```python
from build123d import *

# Parameters (mm, degrees)
SKETCH2_W            = 100
SKETCH2_H            = 100
BOSS_EXTRUDE1_DEPTH  = 5
SKETCH3_W            = 100
SKETCH3_H            = 100
BOSS_EXTRUDE2_DEPTH  = 5
SKETCH8_R            = 5
BOSS_EXTRUDE7_DEPTH  = 30
SKETCH9_W            = 35.4
SKETCH9_H            = 35.4
BOSS_EXTRUDE8_DEPTH  = 20
SKETCH10_W           = 25.4
SKETCH10_H           = 25.4
CUT_EXTRUDE1_DEPTH   = 12.7
BOSS_EXTRUDE21_DEPTH = 10
FILLET14_R           = 4
FILLET13_R           = 4
SKETCH24_W           = 10
SKETCH24_H           = 10
BOSS_EXTRUDE22_DEPTH = 15
BOSS_EXTRUDE25_DEPTH = 10
SKETCH26_W           = 10
SKETCH26_H           = 10
BOSS_EXTRUDE26_DEPTH = 15
FILLET18_R           = 4
FILLET17_R           = 4
BOSS_EXTRUDE23_DEPTH = 10
SKETCH25_W           = 10
SKETCH25_H           = 10
BOSS_EXTRUDE24_DEPTH = 15
FILLET15_R           = 4
FILLET16_R           = 4
BOSS_EXTRUDE10_DEPTH = 10
FILLET19_R           = 4
SKETCH27_W           = 10
SKETCH27_H           = 10
BOSS_EXTRUDE27_DEPTH = 15
FILLET20_R           = 4
SKETCH33_W           = 65
SKETCH33_H           = 65
BOSS_EXTRUDE29_DEPTH = 5
BOSS_EXTRUDE28_DEPTH = 10
BOSS_EXTRUDE32_DEPTH = 10
BOSS_EXTRUDE31_DEPTH = 10
BOSS_EXTRUDE33_DEPTH = 10
BOSS_EXTRUDE34_DEPTH = 10
BOSS_EXTRUDE35_DEPTH = 10
BOSS_EXTRUDE36_DEPTH = 10
BOSS_EXTRUDE37_DEPTH = 10


with BuildPart() as part:
    # Sketch2 → Boss-Extrude1 (new body)
    with BuildSketch(Plane(origin=(0, 0, 0), x_dir=(1, 0, 0), z_dir=(0, 1, 0))):
        Rectangle(SKETCH2_W, SKETCH2_H)
    extrude(amount=BOSS_EXTRUDE1_DEPTH)

    # Sketch3 → Boss-Extrude2 (add)
    with BuildSketch(Plane.XZ):
        Rectangle(SKETCH3_W, SKETCH3_H)
    extrude(amount=BOSS_EXTRUDE2_DEPTH)

    # Sketch8 → Boss-Extrude7 (add)
    with BuildSketch(Plane.XZ.offset(5)):
        with Locations(Location((0, 0, 0), (0, 0, 90))):
            Circle(SKETCH8_R)
    extrude(amount=BOSS_EXTRUDE7_DEPTH)

    # Sketch9 → Boss-Extrude8 (add)
    with BuildSketch(Plane.XZ.offset(35)):
        Rectangle(SKETCH9_W, SKETCH9_H)
    extrude(amount=BOSS_EXTRUDE8_DEPTH)

    # Sketch10 → Cut-Extrude1 (cut)
    with BuildSketch(Plane.XZ.offset(55)):
        Rectangle(SKETCH10_W, SKETCH10_H)
    extrude(amount=-CUT_EXTRUDE1_DEPTH, mode=Mode.SUBTRACT)

    # Sketch11 → Boss-Extrude21 (add)
    with BuildSketch(Plane(origin=(50, 0, 0), x_dir=(0, 0, -1), z_dir=(1, 0, 0))):
        Polygon((5, -5), (5, 12.5), (1, 12.5), (1, 9.5), (3, 5), (-3, 5), (-1, 9.5), (-1, 12.5), (-5, 12.5), (-5, -5), align=None)
    extrude(amount=BOSS_EXTRUDE21_DEPTH)

    # Fillet14
    # the kernel refuses this fillet: 4 mm, written as the material it takes off along each edge
    with BuildSketch(Plane(origin=(40.317541634, 12.5, -1), x_dir=(0, 0, -1), z_dir=(1, 0, 0))) as fillet14_piece_1:
        with BuildLine():
            CenterArc((3.872983346, -4), FILLET14_R, 90, 75.522487814)
            Line((0, -3), (-0.077459667, -2.98))
            ThreePointArc((-0.077459667, -2.98), (-0.08, -1.5), (-0.08, 0))
            Line((-0.08, 0), (0, 0.08))
            Line((0, 0.08), (3.872983346, 0.08))
            Line((3.872983346, 0.08), (3.872983346, 0))
        make_face()
    extrude(amount=29.364916731, mode=Mode.SUBTRACT)

    # Fillet13
    # the kernel refuses this fillet: 4 mm, written as the material it takes off along each edge
    with BuildSketch(Plane(origin=(40.317541634, 12.5, 1), x_dir=(0, 0, 1), z_dir=(1, 0, 0))) as fillet13_piece_1:
        with BuildLine():
            CenterArc((3.872983346, 4), FILLET13_R, 194.477512186, 75.522487814)
            Line((0, 3), (-0.077459667, 2.98))
            ThreePointArc((-0.077459667, 2.98), (-0.08, 1.5), (-0.08, 0))
            Line((-0.08, 0), (0, -0.08))
            Line((0, -0.08), (3.872983346, -0.08))
            Line((3.872983346, -0.08), (3.872983346, 0))
        make_face()
    extrude(amount=29.364916731, mode=Mode.SUBTRACT)

    # Sketch24 → Boss-Extrude22 (add)
    with BuildSketch(Plane(origin=(60, 0, 0), x_dir=(0, 0, -1), z_dir=(1, 0, 0))):
        Rectangle(SKETCH24_W, SKETCH24_H)
    extrude(amount=BOSS_EXTRUDE22_DEPTH)

    # Sketch13 → Boss-Extrude25 (add)
    with BuildSketch(Plane.ZY.offset(50)):
        Polygon((-5, 12.5), (-5, -5), (5, -5), (5, 12.5), (1, 12.5), (1, 9.5), (3, 5), (-3, 5), (-1, 9.5), (-1, 12.5), align=None)
    extrude(amount=BOSS_EXTRUDE25_DEPTH)

    # Sketch26 → Boss-Extrude26 (add)
    with BuildSketch(Plane.ZY.offset(60)):
        Rectangle(SKETCH26_W, SKETCH26_H)
    extrude(amount=BOSS_EXTRUDE26_DEPTH)

    # Fillet18
    # the kernel refuses this fillet: 4 mm, written as the material it takes off along each edge
    with BuildSketch(Plane(origin=(-40.317541634, 12.5, 1), x_dir=(0, 0, 1), z_dir=(-1, 0, 0))) as fillet18_piece_1:
        with BuildLine():
            CenterArc((3.872983346, -4), FILLET18_R, 90, 75.522487814)
            Line((0, -3), (-0.077459667, -2.98))
            ThreePointArc((-0.077459667, -2.98), (-0.08, -1.5), (-0.08, 0))
            Line((-0.08, 0), (0, 0.08))
            Line((0, 0.08), (3.872983346, 0.08))
            Line((3.872983346, 0.08), (3.872983346, 0))
        make_face()
    extrude(amount=29.364916731, mode=Mode.SUBTRACT)

    # Fillet17
    # the kernel refuses this fillet: 4 mm, written as the material it takes off along each edge
    with BuildSketch(Plane(origin=(-40.317541634, 12.5, -1), x_dir=(0, 0, -1), z_dir=(-1, 0, 0))) as fillet17_piece_1:
        with BuildLine():
            CenterArc((3.872983346, 4), FILLET17_R, 194.477512186, 75.522487814)
            Line((0, 3), (-0.077459667, 2.98))
            ThreePointArc((-0.077459667, 2.98), (-0.08, 1.5), (-0.08, 0))
            Line((-0.08, 0), (0, -0.08))
            Line((0, -0.08), (3.872983346, -0.08))
            Line((3.872983346, -0.08), (3.872983346, 0))
        make_face()
    extrude(amount=29.364916731, mode=Mode.SUBTRACT)

    # Sketch14 → Boss-Extrude23 (add)
    with BuildSketch(Plane(origin=(0, 0, -50), x_dir=(-1, 0, 0), z_dir=(0, 0, -1))):
        Polygon((-5, 12.5), (-1, 12.5), (-1, 9.5), (-3, 5), (3, 5), (1, 9.5), (1, 12.5), (5, 12.5), (5, -5), (-5, -5), align=None)
    extrude(amount=BOSS_EXTRUDE23_DEPTH)

    # Sketch25 → Boss-Extrude24 (add)
    with BuildSketch(Plane(origin=(0, 0, -60), x_dir=(-1, 0, 0), z_dir=(0, 0, -1))):
        Rectangle(SKETCH25_W, SKETCH25_H)
    extrude(amount=BOSS_EXTRUDE24_DEPTH)

    # Fillet15
    # the kernel refuses this fillet: 4 mm, written as the material it takes off along each edge
    with BuildSketch(Plane(origin=(-1, 12.5, -40.317541634), x_dir=(0, -1, 0), z_dir=(0, 0, -1))) as fillet15_piece_1:
        with BuildLine():
            CenterArc((4, 3.872983346), FILLET15_R, 180, 75.522487814)
            Line((0, 3.872983346), (-0.08, 3.872983346))
            Line((-0.08, 3.872983346), (-0.08, 0))
            Line((-0.08, 0), (0, -0.08))
            ThreePointArc((0, -0.08), (1.5, -0.08), (2.98, -0.077459667))
            Line((2.98, -0.077459667), (3, 0))
        make_face()
    extrude(amount=29.364916731, mode=Mode.SUBTRACT)

    # Fillet16
    # the kernel refuses this fillet: 4 mm, written as the material it takes off along each edge
    with BuildSketch(Plane(origin=(1, 12.5, -40.317541634), x_dir=(1, 0, 0), z_dir=(0, 0, -1))) as fillet16_piece_1:
        with BuildLine():
            CenterArc((3.872983346, 4), FILLET16_R, 194.477512186, 75.522487814)
            Line((0, 3), (-0.077459667, 2.98))
            ThreePointArc((-0.077459667, 2.98), (-0.08, 1.5), (-0.08, 0))
            Line((-0.08, 0), (0, -0.08))
            Line((0, -0.08), (3.872983346, -0.08))
            Line((3.872983346, -0.08), (3.872983346, 0))
        make_face()
    extrude(amount=29.364916731, mode=Mode.SUBTRACT)

    # Sketch12 → Boss-Extrude10 (add)
    with BuildSketch(Plane.XY.offset(50)):
        Polygon((-5, 12.5), (-5, -5), (5, -5), (5, 12.5), (1, 12.5), (1, 9.5), (3, 5), (-3, 5), (-1, 9.5), (-1, 12.5), align=None)
    extrude(amount=BOSS_EXTRUDE10_DEPTH)

    # Fillet19
    # the kernel refuses this fillet: 4 mm, written as the material it takes off along each edge
    with BuildSketch(Plane(origin=(-1, 12.5, 40.317541634), x_dir=(-1, 0, 0), z_dir=(0, 0, 1))) as fillet19_piece_1:
        with BuildLine():
            CenterArc((3.872983346, 4), FILLET19_R, 194.477512186, 75.522487814)
            Line((0, 3), (-0.077459667, 2.98))
            ThreePointArc((-0.077459667, 2.98), (-0.08, 1.5), (-0.08, 0))
            Line((-0.08, 0), (0, -0.08))
            Line((0, -0.08), (3.872983346, -0.08))
            Line((3.872983346, -0.08), (3.872983346, 0))
        make_face()
    extrude(amount=29.364916731, mode=Mode.SUBTRACT)

    # Sketch27 → Boss-Extrude27 (add)
    with BuildSketch(Plane.XY.offset(60)):
        Rectangle(SKETCH27_W, SKETCH27_H)
    extrude(amount=BOSS_EXTRUDE27_DEPTH)

    # Fillet20
    # the kernel refuses this fillet: 4 mm, written as the material it takes off along each edge
    with BuildSketch(Plane(origin=(1, 12.5, 40.317541634), x_dir=(1, 0, 0), z_dir=(0, 0, 1))) as fillet20_piece_1:
        with BuildLine():
            CenterArc((3.872983346, -4), FILLET20_R, 90, 75.522487814)
            Line((0, -3), (-0.077459667, -2.98))
            ThreePointArc((-0.077459667, -2.98), (-0.08, -1.5), (-0.08, 0))
            Line((-0.08, 0), (0, 0.08))
            Line((0, 0.08), (3.872983346, 0.08))
            Line((3.872983346, 0.08), (3.872983346, 0))
        make_face()
    extrude(amount=29.364916731, mode=Mode.SUBTRACT)

    # Sketch30 → Boss-Extrude28 (add)
    with BuildSketch(Plane.ZY.offset(50)):
        Polygon((-27.5, 5), (-22.5, 5), (-22.5, -5), (-32.5, -5), (-32.5, 5), align=None)
    extrude(amount=BOSS_EXTRUDE28_DEPTH)



with BuildPart() as body_2:
    # Sketch33 → Boss-Extrude29 (new body)
    with BuildSketch(Plane(origin=(0, 85, 0), x_dir=(1, 0, 0), z_dir=(0, 1, 0))):
        Rectangle(SKETCH33_W, SKETCH33_H)
    extrude(amount=-BOSS_EXTRUDE29_DEPTH)


with BuildPart() as part_1:
    add(part.part)

    add(body_2.part)  # Boss-Extrude32 merges body 2
    # Sketch40 → Boss-Extrude32 (add)
    with BuildSketch(Plane(origin=(0, 0, -32.5), x_dir=(-1, 0, 0), z_dir=(0, 0, -1))):
        Polygon((60, 5), (32.5, 80), (22.5, 80), (50, 5), align=None)
    extrude(amount=-BOSS_EXTRUDE32_DEPTH)

    # Sketch37 → Boss-Extrude31 (add)
    with BuildSketch(Plane.XY.offset(50)):
        Polygon((-27.5, 5), (-22.5, 5), (-22.5, -5), (-32.5, -5), (-32.5, 5), align=None)
    extrude(amount=BOSS_EXTRUDE31_DEPTH)

    # Sketch41 → Boss-Extrude33 (add)
    with BuildSketch(Plane.ZY.offset(32.5)):
        Polygon((60, 5), (32.5, 80), (22.5, 80), (50, 5), align=None)
    extrude(amount=-BOSS_EXTRUDE33_DEPTH)

    # Sketch42 → Boss-Extrude34 (add)
    with BuildSketch(Plane(origin=(50, 0, 0), x_dir=(0, 0, -1), z_dir=(1, 0, 0))):
        Polygon((-27.5, 5), (-22.5, 5), (-22.5, -5), (-32.5, -5), (-32.5, 5), align=None)
    extrude(amount=BOSS_EXTRUDE34_DEPTH)

    # Sketch43 → Boss-Extrude35 (add)
    with BuildSketch(Plane.XY.offset(32.5)):
        Polygon((32.5, 80), (60, 5), (50, 5), (22.5, 80), align=None)
    extrude(amount=-BOSS_EXTRUDE35_DEPTH)

    # Sketch44 → Boss-Extrude36 (add)
    with BuildSketch(Plane(origin=(0, 0, -50), x_dir=(-1, 0, 0), z_dir=(0, 0, -1))):
        Polygon((-27.5, 5), (-22.5, 5), (-22.5, -5), (-32.5, -5), (-32.5, 5), align=None)
    extrude(amount=BOSS_EXTRUDE36_DEPTH)

    # Sketch45 → Boss-Extrude37 (add)
    with BuildSketch(Plane(origin=(32.5, 0, 0), x_dir=(0, 0, -1), z_dir=(1, 0, 0))):
        Polygon((32.5, 80), (60, 5), (50, 5), (22.5, 80), align=None)
    extrude(amount=-BOSS_EXTRUDE37_DEPTH)


solid = part_1.part
```
Check sheet for the modelled part. Datum: model origin and axes. Units: mm. A direction names the side the tool comes from. Round coordinates to 2 decimals unless told otherwise and drop trailing zeros. Write each loop counter-clockwise with the first axis right and the second up, starting at its lowest first coordinate (ties: lowest second). Pieces come first, ordered by that corner, then holes. Notation, with made-up numbers: (31, -2) -> (87, -2) arc R17 cw to (87, 15) -> close; hole circle Ø6 at (78, 86.25). An arc over 180 degrees is marked (long way). One line per question, with ' | ' between items. Start each with the question number.
1. Set-up check for faces 1 (the face through (3, 9, -60)), 2 (the face through (36.44, 41.98, 27.57)), 3 (the face through (12.7, -49, 0)), 4 (the face through (60, 9, -3)), 5 (the face through (-50, 0, 27)): record each of +Z, -Z, +X, -X, +Y, -Y from which the full face is reachable in a straight line by a thin tool's end or side.
2. Sectioned sample at A-A, the plane z = -45. Record the cut outline in (x, y), then the cut area to 3 significant figures.
3. Scan lines: line 1 along Y through (x, z) = (16.5, 3.5); line 2 along Y through (x, z) = (19, -6); line 3 along Z through (x, y) = (-57, 7). Record each from-to range of solid material in increasing order. Write a range as from..to.
4. Release check for a two-part mould opening along X. For faces 6 (the face through (-60, 9, 3)), 7 (the face through (2.453, 11.685, 54.93)), 8 (the face through (46.06, 43.02, 27.57)) record: +X half, -X half, draft (parallel to the pull), parting line (faces both ways), or undercut.
5. Depth check by flat-ended pin: pin 1 (14 mm diameter, centred on y = 0.5, z = -64, fed in from -X); pin 2 (2 mm diameter, centred on x = 34, z = 50.5, fed in from -Y); pin 3 (12 mm diameter, centred on x = -53, y = -13.5, fed in from -Z); pin 4 (6.5 mm diameter, centred on y = -46.5, z = 0.5, fed in from +X). Enter the tip coordinate at first touch or a pass-through.
6. Sectioned sample at B-B, the plane x = -35.5. Record the cut outline in (y, z), then the cut area to 3 significant figures.
7. Sectioned sample at C-C, the plane z = -25. Record the cut outline in (x, y).
Taken from the geometry:
1) face 1: -Z, +X, -X, +Y | face 2: +Z | face 3: -Y | face 4: +Z, -Z, +X, +Y | face 5: +Z, -X, +Y, -Y
2) outline: (-50, -5) -> (50, -5) -> (50, 5) -> (-50, 5) -> close; (22.5, 18.64) -> (32.5, 18.64) -> (32.5, 45.91) -> (22.5, 45.91) -> close | area: 1,270 mm^2
3) line 1: y = -55..-35, -5..5, 80..85 | line 2: y = -5..5, 80..85 | line 3: z = -32.5..-22.5, -5..-2.11, 2.11..5
4) face 6: -X half | face 7: undercut | face 8: +X half
5) pin 1: stops at x = -5 | pin 2: stops at y = -5 | pin 3: passes through | pin 4: stops at x = 17.7
6) outline: (-5, -50) -> (5, -50) -> (5, 50) -> (-5, 50) -> close; (44.55, -32.5) -> (71.82, -32.5) -> (71.82, -22.5) -> (44.55, -22.5) -> close | area: 1,270 mm^2
7) outline: (-60, -5) -> (50, -5) -> (50, 5) -> (-50, 5) -> (-22.5, 80) -> (22.5, 80) -> (22.5, 73.18) -> (32.5, 73.18) -> (32.5, 85) -> (-32.5, 85) -> (-32.5, 80) -> (-60, 5) -> close
